The figure shows three views and two pictorial views of one solid part (mm, origin at its lowest corner). Answer the questions. Coordinates: 2 decimals unless noted, no trailing zeros. Order: outer loops, then holes, each group sorted by start corner. A loop starts at its lowest first (then second) coordinate and runs counter-clockwise, first axis right, second up. Notation, with made-up numbers: (88, 51) - (101, 51) arc R16 cw to (101, 58) - close; hole circle Ø4 at (76.25, -26.5). An arc over 180 degrees is marked (long way). Answer as a JSON object with one key per item and string values. Group by question number.
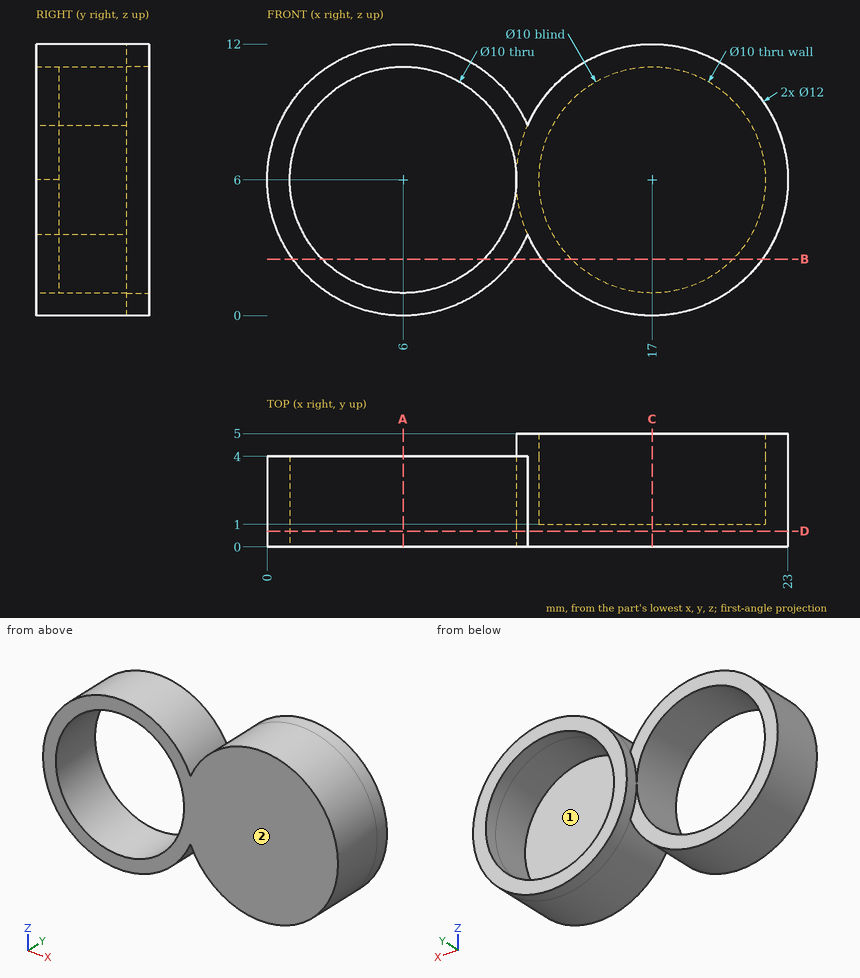
1. A cutting plane is placed at D-D on y = 0.7. Write down the section's boundary in (x, z), and give its area (3 significant figures).
2. A cutting plane is placed at B-B on z = 2.5. Write down the section's boundary in (x, y), and give its area (3 significant figures).
3. Given pin 1 (1.5 mm diameter, centred on x = 4.5, y = 4.5, fed in from -Z); pin 2 (1 mm diameter, centred on x = 15.5, y = 4, fed in from +Z); pin 3 (4 mm diameter, centred on x = 11, z = 8, fed in from +Y); pin 4 (6 mm diameter, centred on x = 5.5, z = 9, fed in from +Y), each flat-ended and moving along its own axis, determine where each tip first touches the part or whether it passes through.
4. For a pull along X with two mould halves and no side action, classify the marked faces 1 and 2 as pulls with the +X half, pulls with the -X half, needs draft (parallel to the pull), parting line crosses it, or undercut.
5. Straight lines are drawn through the part: L1, parallel to Z at x = 6, y = 1.75; L2, parallel to X at y = 1.95, z = 9.25; L3, parallel to X at y = 2.55, z = 6.5. For each, find the intervals that lie inside material, in ascending order.
6. A cutting plane is placed at C-C on x = 17. Write down the section's boundary in (y, z), and give its area (3 significant figures).
7. A cutting plane is placed at A-A on x = 6. Write down the section's boundary in (y, z), and give its area (3 significant figures).
Derived:
{
 "1": {"outline": "(11.5, 3.6) arc R6 ccw (long way) to (11.5, 8.4) arc R6 ccw (long way) to start; hole circle Ø10 at (6, 6)", "area": "144 mm2"},
 "2": {"outline": "(1.13, 0) - (2.43, 0) - (2.43, 4) - (1.13, 4) - close; (9.57, 0) - (10.87, 0) - (10.87, 4) - (9.57, 4) - close; (12.13, 0) - (21.87, 0) - (21.87, 5) - (20.57, 5) - (20.57, 1) - (13.43, 1) - (13.43, 5) - (12.13, 5) - close", "area": "30.6 mm2"},
 "3": {"pin 1": "stops at z = 0.07", "pin 2": "stops at z = 11.92", "pin 3": "stops at y = 5", "pin 4": "stops at y = 4"},
 "4": {"face 1": "undercut", "face 2": "needs draft"},
 "5": {"L1": "z = 0 to 1, 11 to 12", "L2": "x = 0.96 to 2.2, 9.8 to 11.04, 11.96 to 13.2, 20.8 to 22.04", "L3": "x = 0.02 to 1.03, 10.97 to 12.03, 21.97 to 22.98"},
 "6": {"outline": "(0, 0) - (5, 0) - (5, 1) - (1, 1) - (1, 11) - (5, 11) - (5, 12) - (0, 12) - close", "area": "20.0 mm2"},
 "7": {"outline": "(0, 0) - (4, 0) - (4, 1) - (0, 1) - close; (0, 11) - (4, 11) - (4, 12) - (0, 12) - close", "area": "8.00 mm2"}
}
